Geometry: see drawing. Coordinates: mm, zero at the bounding-box minimum. A direction names the side the tool comes from. Round coordinates to 2 decimals unless told otherwise and drop trailing zeros. Order: outer loops, then holes, each group sorted by start corner. A loop starts at its lowest first (then second) coordinate and runs counter-clockwise, first axis right, second up. Notation, with made-up numbers: (11, 5) -> (41, 5) arc R19 ccw to (41, 37) -> close; hole circle Ø1 at (28, -33.5). An arc over 180 degrees is marked (long way). Use a Markdown table: item, result.
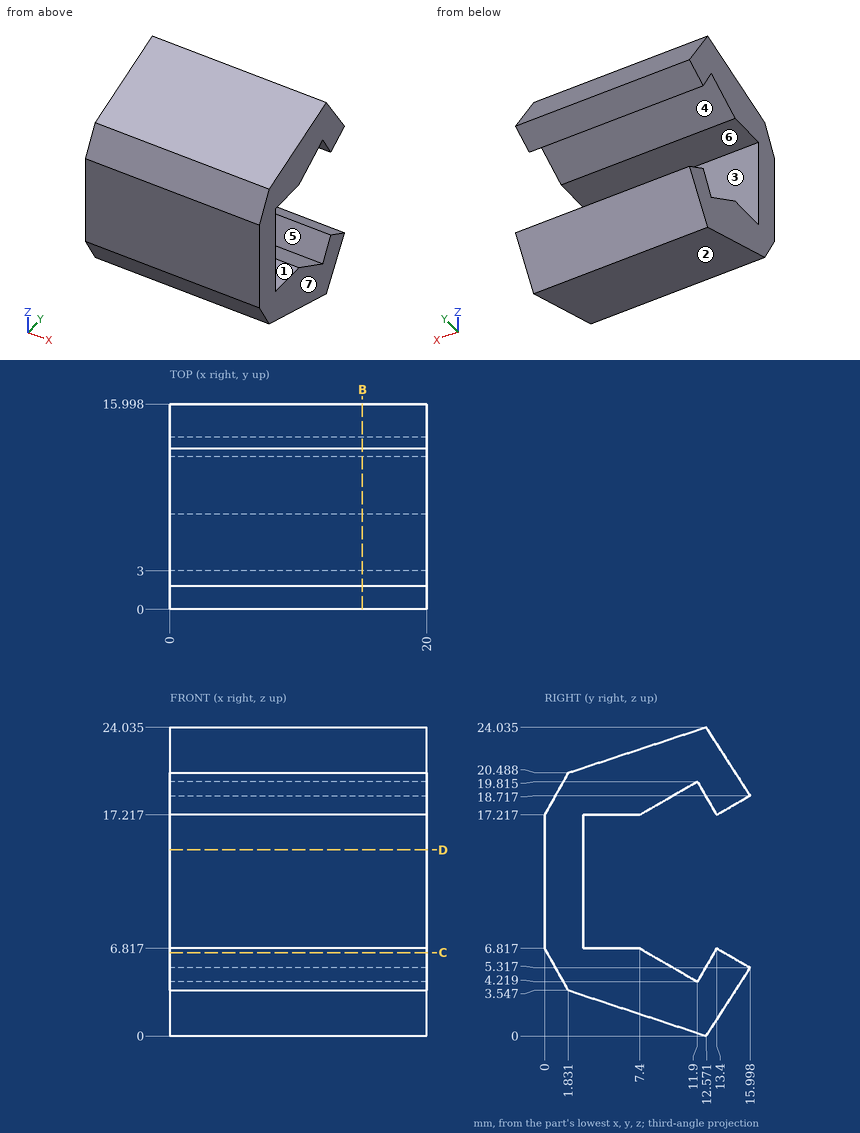
1) Set-up query: the marked faces 5, 6 and 7. Return all of +Z, -Z, +X, -X, +Y, -Y with unobstructed straight access to the full face (end or side cutting, diameter ignored); none if empty.
Answer key:
| item | result |
|---|---|
| face 5 | +X, -X |
| face 6 | +X, -X, +Y |
| face 7 | +Z, -Z, +X, +Y, -Y |
2) Cut plane D-D on z = 14.5. Return loops of the section in (x, y), and give its area (3 significant figures).
Answer key:
| item | result |
|---|---|
| outline | (0, 0) -> (20, 0) -> (20, 3) -> (0, 3) -> close |
| area | 60.0 mm^2 |
3) Cut plane B-B on x = 15. Return loops of the section in (y, z) (1 decimal).
Answer key:
| item | result |
|---|---|
| outline | (0, 6.8) -> (1.8, 3.5) -> (12.6, 0) -> (16, 5.3) -> (13.4, 6.8) -> (11.9, 4.2) -> (7.4, 6.8) -> (3, 6.8) -> (3, 17.2) -> (7.4, 17.2) -> (11.9, 19.8) -> (13.4, 17.2) -> (16, 18.7) -> (12.6, 24) -> (1.8, 20.5) -> (0, 17.2) -> close |
4) Ray query, probe 1 along Y at (x, z) = (17, 11.75); probe 2 along Z at (x, y) = (15.75, 7) (1 decimal); probe 3 along Z at (x, y) = (2.75, 6.5) (1 decimal). Return the intervals inside material, ascending.
Answer key:
| item | result |
|---|---|
| probe 1 | y = 0 to 3 |
| probe 2 | z = 1.8 to 6.8, 17.2 to 22.2 |
| probe 3 | z = 2 to 6.8, 17.2 to 22 |
5) Contact query for flat-ended pins moving along their axis: P1, Ø1, axis at x = 6.5, y = 6, coming from the -Z side (1 decimal); P2, Ø2, axis at x = 10, y = 6, coming from the +Z side (1 decimal); P3, Ø8.5, axis at x = 10.5, z = 10.5, coming from the +Y side (1 decimal). Output: stop coordinate, or through.
Answer key:
| item | result |
|---|---|
| P1 | stops at z = 2 |
| P2 | stops at z = 22.2 |
| P3 | stops at y = 14.4 |
6) Cut plane C-C on z = 6.5. Return loops of the section in (x, y), and give its area (3 significant figures).
Answer key:
| item | result |
|---|---|
| outline | (0, 0.18) -> (20, 0.18) -> (20, 7.95) -> (0, 7.95) -> close; (0, 13.22) -> (20, 13.22) -> (20, 13.95) -> (0, 13.95) -> close |
| area | 170 mm^2 |
7) Draft query along Y for the marked faces 1, 2, 3 and 4. Return one class per face: released by +Y, released by -Y, zero draft, split by the parting line, or undercut.
Answer key:
| item | result |
|---|---|
| face 1 | zero draft |
| face 2 | released by -Y |
| face 3 | released by +Y |
| face 4 | undercut |
